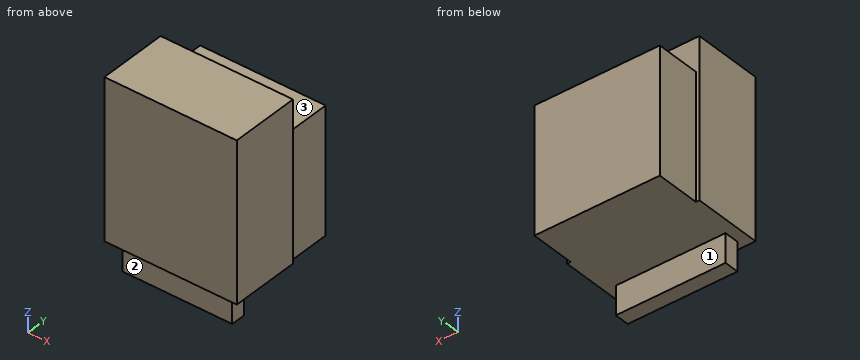
```python
from build123d import *

# Parameters (mm, degrees)
SCHIZZO1_W                   = 31.57
SCHIZZO1_H                   = 37.74
ESTRUSIONE_ESTRUSIONE1_DEPTH = 16.55
SCHIZZO2_W                   = 29.9
SCHIZZO2_H                   = 29.9
ESTRUSIONE_ESTRUSIONE2_DEPTH = 10.63
ESTRUSIONE_ESTRUSIONE3_START = -2
SCHIZZO3_W                   = 26.14
SCHIZZO3_H                   = 6.84
ESTRUSIONE_ESTRUSIONE3_DEPTH = 3.5


with BuildPart() as part:
    # Schizzo1 → Estrusione-Estrusione1 (new body)
    with BuildSketch(Plane(origin=(0, 0, 0), x_dir=(1, 0, 0), z_dir=(0, 1, 0))):
        Rectangle(SCHIZZO1_W, SCHIZZO1_H)
    extrude(amount=ESTRUSIONE_ESTRUSIONE1_DEPTH)

    # Schizzo2 → Estrusione-Estrusione2 (add)
    with BuildSketch(Plane(origin=(0, 16.55, 0), x_dir=(1, 0, 0), z_dir=(0, 1, 0))):
        with Locations((0, 3.92)):
            Rectangle(SCHIZZO2_W, SCHIZZO2_H)
    extrude(amount=ESTRUSIONE_ESTRUSIONE2_DEPTH)

    # Schizzo3 → Estrusione-Estrusione3 (add)
    with BuildSketch(Plane.XZ.offset(ESTRUSIONE_ESTRUSIONE3_START)):
        with Locations((0, -22.29)):
            Rectangle(SCHIZZO3_W, SCHIZZO3_H)
    extrude(amount=-ESTRUSIONE_ESTRUSIONE3_DEPTH)


solid = part.part
```
Part model, mm, in its own coordinate system. Face numbers are marked on the shaded views. A direction names the side the tool comes from. Round coordinates to 2 decimals unless told otherwise and drop trailing zeros. Order: outer loops, then holes, each group sorted by start corner. A loop starts at its lowest first (then second) coordinate and runs counter-clockwise, first axis right, second up. Notation, with made-up numbers: M -36.75,73 L 20.25,73 A21 cw 20.25,83 Z; hole C 60,26.5 d8. An arc over 180 degrees is marked long. Answer in a Markdown table with one row per item. Add a question column.
Q1. Wall check: L1, parallel to X at y = 21, z = -2.5; L2, parallel to Z at x = -10.5, y = 23.5; L3, parallel to Z at x = 1, y = 12. Give the ranges that are in metal, low to high. Write a range as from..to.
Q2. Cut at A-A on z = -7. Give the cut face in (x, y) (3 decimals).
Q3. Cut at B-B on x = 7. Give the cut face in (y, z).
Q4. Cut at D-D on y = 6. Give the cut face in (x, z) (3 decimals), and give its area (3 significant figures).
Q5. Cut at C-C on y = 22. Give the cut face in (x, z), and give its area (3 significant figures).
Q6. 3-axis set-ups, long thin cutter, end or side, ignore diameter. For the marked faces 1, 2 and 3: which of +Z, -Z, +X, -X, +Y, -Y reach the whole face in a straight line?
Q7. Pin check, flat tips, straight feed: pin 1 (8.5 mm diameter, centred on x = -6, y = 24, fed in from +Z); pin 2 (3 mm diameter, centred on y = 3.5, z = -22.5, fed in from +X); pin 3 (3 mm diameter, centred on y = 20, z = -9, fed in from +X). Stop position of each tip, or through.
Established:
| question | item | result |
|---|---|---|
| 1 | L1 | x = -14.95..14.95 |
| 1 | L2 | z = -18.87..11.03 |
| 1 | L3 | z = -18.87..18.87 |
| 2 | outline | M -15.785,0 L 15.785,0 L 15.785,16.55 L 14.95,16.55 L 14.95,27.18 L -14.95,27.18 L -14.95,16.55 L -15.785,16.55 Z |
| 3 | outline | M 0,-18.87 L 2,-18.87 L 2,-25.71 L 5.5,-25.71 L 5.5,-18.87 L 27.18,-18.87 L 27.18,11.03 L 16.55,11.03 L 16.55,18.87 L 0,18.87 Z |
| 4 | outline | M -15.785,-18.87 L 15.785,-18.87 L 15.785,18.87 L -15.785,18.87 Z |
| 4 | area | 1,190 mm2 |
| 5 | outline | M -14.95,-18.87 L 14.95,-18.87 L 14.95,11.03 L -14.95,11.03 Z |
| 5 | area | 894 mm2 |
| 6 | face 1 | -Z, +X, -X, +Y |
| 6 | face 2 | -Z, +X, -X, -Y |
| 6 | face 3 | +Z, +X, -X, +Y |
| 7 | pin 1 | stops at z = 11.03 |
| 7 | pin 2 | stops at x = 13.07 |
| 7 | pin 3 | stops at x = 14.95 |
